Could you check a few things on this model? Use its own coordinates, in mm. Round coordinates to 2 decimals unless told otherwise and drop trailing zeros. Write each loop counter-clockwise with the first axis right and the second up, starting at its lowest first coordinate (ties: lowest second). Pieces come first, ordered by that corner, then holes. Notation, with made-up numbers: (81, 51.5) - (113, 51.5) arc R23 ccw to (113, 62.5) - close; hole circle Ø4 at (-7, 36). An arc over 180 degrees is marked (long way). Write each question's results on one line, items separated by ' | '. Start each with the question number.
(1) Imagine slicing it at A-A on z = 2.45. Write out the boundary of the cut face in (x, y), then the cut area to 3 significant figures.
(2) Please list where these lines run through material, in increasing order: line 1 (X direction, y = -13, z = 0.65); line 2 (Y direction, x = 6, z = 2.6); line 3 (X direction, y = -10.5, z = 2.85). Write a range as [from, to].
(3) Imagine slicing it at B-B on x = 1.5. Write out the boundary of the cut face in (y, z), then the cut area to 3 significant figures.
```python
from build123d import *

# Parameters (mm, degrees)
SKETCH1_W           = 32.526911934
SKETCH1_H           = 32.526911934
BOSS_EXTRUDE1_DEPTH = 4
FILLET1_R           = 4
CHAMFER1_SIZE       = 2


with BuildPart() as part:
    # Sketch1 → Boss-Extrude1 (new body)
    with BuildSketch(Plane.XY):
        Rectangle(SKETCH1_W, SKETCH1_H)
    extrude(amount=BOSS_EXTRUDE1_DEPTH)

    # Fillet1
    fillet1_edges = [part.edges().sort_by_distance(p)[0] for p in [
        (-16.263455967, 16.263455967, 2),
        (16.263455967, 16.263455967, 2),
        (16.263455967, -16.263455967, 2),
        (-16.263455967, -16.263455967, 2),
    ]]
    fillet(fillet1_edges, radius=FILLET1_R)

    # Chamfer1
    chamfer1_edges = [part.edges().sort_by_distance(p)[0] for p in [
        (0, -16.263455967, 4),
        (-16.263455967, 0, 4),
        (16.263455967, 0, 4),
        (0, 16.263455967, 4),
        (-15.091883092, 15.091883092, 4),
        (15.091883092, 15.091883092, 4),
        (15.091883092, -15.091883092, 4),
        (-15.091883092, -15.091883092, 4),
    ]]
    chamfer(chamfer1_edges, length=CHAMFER1_SIZE)


solid = part.part
```
Response:
1) outline: (-15.81, -12.26) arc R3.55 ccw to (-12.26, -15.81) - (12.26, -15.81) arc R3.55 ccw to (15.81, -12.26) - (15.81, 12.26) arc R3.55 ccw to (12.26, 15.81) - (-12.26, 15.81) arc R3.55 ccw to (-15.81, 12.26) - close | area: 989 mm²
2) line 1: [-16.2, 16.2] | line 2: [-15.66, 15.66] | line 3: [-15.41, 15.41]
3) outline: (-16.26, 0) - (16.26, 0) - (16.26, 2) - (14.26, 4) - (-14.26, 4) - (-16.26, 2) - close | area: 126 mm²
